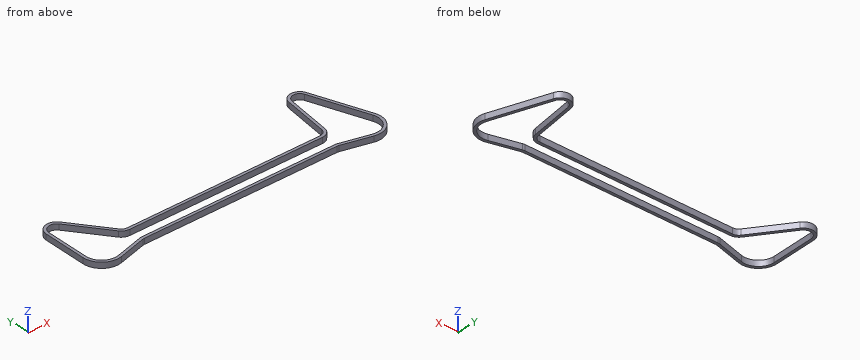
Solid Edge part; units mm, degrees
sketch "Sketch1" plane through (0, 0, 0) normal (0, 0, 1) x (1, 0, 0)
  line L0 (165, -7) -> (25, -7)
  arc A0 (25, -7) -> (23.72, -7.1666) centre (25, -12) ccw
  line L1 (23.72, -7.1666) -> (3.3279, -12.5668)
  arc A1 (3.3279, -12.5668) -> (-12.992, 0.4565) centre (0, 0) cw
  line L2 (-12.992, 0.4565) -> (-11.8954, 31.6634)
  arc A2 (-11.8954, 31.6634) -> (1.6834, 35.7866) centre (-4.4, 31.4) cw
  line L3 (1.6834, 35.7866) -> (20.9444, 9.0756)
  arc A3 (20.9444, 9.0756) -> (25, 7) centre (25, 12) ccw
  line L4 (25, 7) -> (165, 7)
  arc A4 (165, 7) -> (169.9356, 11.2) centre (165, 12) ccw
  line L5 (169.9356, 11.2) -> (175.1902, 43.6199)
  arc A5 (175.1902, 43.6199) -> (188.7379, 44.7221) centre (182.1, 42.5) cw
  line L6 (188.7379, 44.7221) -> (202.3276, 4.1268)
  arc A6 (202.3276, 4.1268) -> (186.6721, -12.5668) centre (190, 0) cw
  line L7 (186.6721, -12.5668) -> (166.28, -7.1666)
  arc A7 (166.28, -7.1666) -> (165, -7) centre (165, -12) ccw
  line L8 (165, -5) -> (25, -5)
  arc A8 (25, -5) -> (23.208, -5.2333) centre (25, -12) ccw
  line L9 (23.208, -5.2333) -> (2.8159, -10.6335)
  arc A9 (2.8159, -10.6335) -> (-10.9932, 0.3863) centre (0, 0) cw
  line L10 (-10.9932, 0.3863) -> (-9.8966, 31.5932)
  arc A10 (-9.8966, 31.5932) -> (0.0611, 34.6169) centre (-4.4, 31.4) cw
  line L11 (0.0611, 34.6169) -> (19.3222, 7.9058)
  arc A11 (19.3222, 7.9058) -> (25, 5) centre (25, 12) ccw
  line L12 (25, 5) -> (165, 5)
  arc A12 (165, 5) -> (171.9098, 10.8801) centre (165, 12) ccw
  line L13 (171.9098, 10.8801) -> (177.1644, 43.3)
  arc A13 (177.1644, 43.3) -> (186.8414, 44.0872) centre (182.1, 42.5) cw
  line L14 (186.8414, 44.0872) -> (200.431, 3.4919)
  arc A14 (200.431, 3.4919) -> (187.1841, -10.6335) centre (190, 0) cw
  line L15 (187.1841, -10.6335) -> (166.792, -5.2333)
  arc A15 (166.792, -5.2333) -> (165, -5) centre (165, -12) ccw
extrude "Protrusion1" add sketch "Sketch1" along normal blind 4
properties material "Steel"
CAD build for the part. Positions are in the model's coordinates, mm. Round coordinates to 2 decimals unless told otherwise and drop trailing zeros. Order: outer loops, then holes, each group sorted by start corner. A loop starts at its lowest first (then second) coordinate and runs counter-clockwise, first axis right, second up.
Item 1: Probe line 1 along Y through (x, z) = (155, 1.05); line 2 along X through (y, z) = (8, 2.15); line 3 along X through (y, z) = (6.5, 1.65). List the from-to ranges inside material, lowest first.
Item 2: Saw through at C-C on y = 41. Write the cut outline in (x, z).
Item 3: Saw through at D-D on y = 26.5. Write the cut outline in (x, z), then the cut area to 3 significant figures.
Item 4: Saw through at A-A on x = 145.5. Write the cut outline in (y, z), then the cut area to 3 significant figures.
Item 5: Pin check, flat tips, straight feed: pin 1 (2 mm diameter, centred on x = 101.5, z = 2.5, fed in from -Y); pin 2 (4 mm diameter, centred on x = 135, y = -2, fed in from -Z); pin 3 (2 mm diameter, centred on x = 82, z = 1.5, fed in from +Y). Stop position of each tip, or through.
Reported:
1. line 1: y = -7 to -5, 5 to 7
1. line 2: x = -12.73 to -10.73, 19.25 to 22, 168 to 170.74, 198.92 to 201.03
1. line 3: x = -12.78 to -10.78, 20.67 to 169.33, 199.42 to 201.53
2. outline: (174.77, 0) - (176.79, 0) - (176.79, 4) - (174.77, 4) - close; (187.87, 0) - (189.98, 0) - (189.98, 4) - (187.87, 4) - close
3. outline: (-12.08, 0) - (-10.08, 0) - (-10.08, 4) - (-12.08, 4) - close; (5.91, 0) - (8.38, 0) - (8.38, 4) - (5.91, 4) - close; (172.42, 0) - (174.44, 0) - (174.44, 4) - (172.42, 4) - close; (192.73, 0) - (194.84, 0) - (194.84, 4) - (192.73, 4) - close
3. area: 34.4 mm2
4. outline: (-7, 0) - (-5, 0) - (-5, 4) - (-7, 4) - close; (5, 0) - (7, 0) - (7, 4) - (5, 4) - close
4. area: 16.0 mm2
5. pin 1: stops at y = -7
5. pin 2: passes through
5. pin 3: stops at y = 7
